from build123d import *

# Parameters (mm, degrees)
F1_DEPTH  = 35
F2_R      = 3
F3_DEPTH  = 34.3740698971
F4_R      = 5
F5_DEPTH  = 120.001
F6_R      = 11.25
F7_DEPTH  = 7.5
F8_R      = 11.25
F9_DEPTH  = 7.5
F10_R     = 11.25
F11_DEPTH = 47.5
F12_R     = 11.25
F13_DEPTH = 47.5


with BuildPart() as f1:
    # F0 (on Front) → F1 (new body)
    with BuildSketch(Plane.XZ):
        with BuildLine():
            Line((-40, 19.3730698971), (-60, 5))
            Line((-60, 5), (-60, 0))
            Line((-60, 0), (-60, -55))
            Line((-60, -55), (-40, -55))
            Line((-40, -55), (-30, -15))
            Line((-30, -15), (0, -15))
            Line((0, -15), (30, -15))
            Line((30, -15), (40, -55))
            Line((40, -55), (60, -55))
            Line((60, -55), (60, 0))
            Line((60, 0), (60, 5))
            Line((60, 5), (40, 19.3730698971))
            Line((40, 19.3730698971), (10, 19.3730698971))
            ThreePointArc((10, 19.3730698971), (0, 9.3730698971), (-10, 19.3730698971))
            Line((-10, 19.3730698971), (-40, 19.3730698971))
        make_face()
    extrude(amount=F1_DEPTH)

    # F2 (on face) → F3 (cut, through all)
    with BuildSketch(Plane(origin=(0, 0, -15), x_dir=(1, 0, 0), z_dir=(0, 0, -1))):
        with Locations((-16.9, 17.5)):
            Circle(F2_R)
        with Locations((16.9, 17.5)):
            Circle(F2_R)
    extrude(amount=-F3_DEPTH, mode=Mode.SUBTRACT)

    # F4 (on face) → F5 (cut, through all)
    with BuildSketch(Plane(origin=(-60, 0, 0), x_dir=(0, -1, 0), z_dir=(-1, 0, 0))):
        with Locations((17.5, -40)):
            Circle(F4_R)
    extrude(amount=-F5_DEPTH, mode=Mode.SUBTRACT)

    # F6 (on face) → F7 (cut)
    with BuildSketch(Plane(origin=(-60, 0, 0), x_dir=(0, -1, 0), z_dir=(-1, 0, 0))):
        with Locations((17.5, -40)):
            Circle(F6_R)
    extrude(amount=-F7_DEPTH, mode=Mode.SUBTRACT)

    # F8 (on face) → F9 (cut)
    with BuildSketch(Plane.YZ.offset(60)):
        with Locations((-17.5, -40)):
            Circle(F8_R)
    extrude(amount=-F9_DEPTH, mode=Mode.SUBTRACT)

    # F10 (on Right) → F11 (cut)
    with BuildSketch(Plane.YZ):
        with Locations((-17.5, -40)):
            Circle(F10_R)
    extrude(amount=-F11_DEPTH, mode=Mode.SUBTRACT)

    # F12 (on Right) → F13 (cut)
    with BuildSketch(Plane.YZ):
        with Locations((-17.5, -40)):
            Circle(F12_R)
    extrude(amount=F13_DEPTH, mode=Mode.SUBTRACT)


solid = f1.part
Input: part model. Units: mm. Frame: model coordinates. A direction names the side the tool comes from. Coordinates: 2 decimals unless noted, no trailing zeros. Loops run counter-clockwise (first coordinate to the right, second up) from the corner with the lowest first, then second, coordinate; pieces in that order, holes last. Notation, with made-up numbers: (-0.75, 2.5) - (9.25, 2.5) arc R22 ccw to (9.25, 11.5) - close; hole circle Ø3 at (67, -32). An arc over 180 degrees is marked (long way). Answer in a Markdown table with one row per item. Add a question column.
Item 1: Contact query for flat-ended pins moving along their axis: P1, Ø5.5, axis at x = -16.9, y = -17.5, coming from the -Z side; P2, Ø1.5, axis at x = 11.5, y = -14, coming from the -Z side; P3, Ø18, axis at y = -17.5, z = -40, coming from the +X side; P4, Ø11.5, axis at y = -17.5, z = -40, coming from the -X side. Output: stop coordinate, or through.
Item 2: Section query C-C on y = -8. Return the cut outline in (x, z), then the cut area to 3 significant figures.
Item 3: Mould query, pull axis Z, two halves, no side actions, for faces 1 (the cylindrical face through (-56.302, -16.035, -28.846)), 2 (the flat face through (60, -17, -25)), 3 (the flat face through (-50, -17, -55)), 4 (the flat face through (47.5, -15, -45)). Classes: released by +Z, released by -Z, zero draft, split by the parting line, or undercut.
Item 4: Access query for faces 5 (the flat face through (-47.5, -15, -45)), 6 (the flat face through (0, -17, -15)), 7 (the flat face through (-52.5, -20, -45)), 8 (the cylindrical face through (56.302, -18.965, -28.846)). Directions: +Z, -Z, +X, -X, +Y, -Y. A direction counts if a zero-diameter tool reaches every point of the face in a straight line with its end or side. Return the directions, or none.
Item 5: Line query: line 1 along Y through (x, z) = (-42, -40); line 2 along Y through (x, z) = (16.9, 0.5); line 3 along X through (y, z) = (-17.5, 8.5). Output: solid intervals per line, ascending. Write a range as [from, to].
Item 6: Section query B-B on x = 16.9. Return the cut outline in (y, z).
Item 7: Section query D-D on x = -38.5. Return the cut outline in (y, z), then the cut area to 3 significant figures.
Item 8: Section query A-A on z = -40. State how many separate pieces and enclosed holes the cut face has, then the cut area to 3 significant figures.
Recorded:
| question | item | result |
|---|---|---|
| 1 | P1 | through |
| 1 | P2 | z = -15 |
| 1 | P3 | x = 52.5 |
| 1 | P4 | x = -52.5 |
| 2 | outline | (-60, -55) - (-40, -55) - (-37.76, -46.03) - (-47.5, -46.03) - (-47.5, -33.97) - (-34.74, -33.97) - (-30, -15) - (30, -15) - (34.74, -33.97) - (47.5, -33.97) - (47.5, -46.03) - (37.76, -46.03) - (40, -55) - (60, -55) - (60, -46.03) - (52.5, -46.03) - (52.5, -33.97) - (60, -33.97) - (60, 5) - (40, 19.37) - (10, 19.37) arc R10 cw to (-10, 19.37) - (-40, 19.37) - (-60, 5) - (-60, -33.97) - (-52.5, -33.97) - (-52.5, -46.03) - (-60, -46.03) - close |
| 2 | area | 5,230 mm^2 |
| 3 | face 1 | undercut |
| 3 | face 2 | zero draft |
| 3 | face 3 | released by -Z |
| 3 | face 4 | undercut |
| 4 | face 5 | none |
| 4 | face 6 | -Z, +Y, -Y |
| 4 | face 7 | -X |
| 4 | face 8 | +X |
| 5 | line 1 | [-35, -28.75], [-6.25, 0] |
| 5 | line 2 | [-35, -20.5], [-14.5, 0] |
| 5 | line 3 | [-55.13, -19.9], [-13.9, 13.9], [19.9, 55.13] |
| 6 | outline | (-35, -15) - (-20.5, -15) - (-20.5, 19.37) - (-35, 19.37) - close; (-14.5, -15) - (0, -15) - (0, 19.37) - (-14.5, 19.37) - close |
| 7 | outline | (-35, -49) - (-24.25, -49) arc R11.25 cw (long way) to (-10.75, -49) - (0, -49) - (0, 19.37) - (-35, 19.37) - close |
| 7 | area | 2,020 mm^2 |
| 8 | separate pieces | 4 |
| 8 | enclosed holes | 0 |
| 8 | area | 719 mm^2 |
